The model under review builds one solid part; all positions refer to its coordinate system, in mm. A direction names the side the tool comes from. Coordinates: 2 decimals unless noted, no trailing zeros. Write each loop counter-clockwise with the first axis right and the second up, starting at its lowest first coordinate (ties: lowest second). Pieces come first, ordered by that corner, then holes. Notation, with made-up numbers: (-39, 49.25) - (-15, 49.25) arc R19 ccw to (-15, 83.25) - close; hole circle Ø9 at (7, 18.5). An arc over 180 degrees is marked (long way). Answer as CSV lines item,"result". Start each with the question number.
```python
from build123d import *

# Parameters (mm, degrees)
SKETCH_3_R          = 2.075
CUT_EXTRUDE_1_DEPTH = 60
FILLET_1_R          = 1


with BuildPart() as part:
    # 草图2 → 旋转1 (revolve)
    with BuildSketch(Plane.XY, mode=Mode.PRIVATE) as revolve_1_sk:
        Polygon((0, 0), (0, 50), (-15, 50), (-12, 25), (-15, 0), align=None)
    revolve(revolve_1_sk.sketch.rotate(Axis((0, 0, 0), (0, 1, 0)), 180), axis=Axis((0, 0, 0), (0, 1, 0)))

    # 草图3 → 切除-拉伸1 (cut)
    with BuildSketch(Plane.XZ):
        with Locations(Location((0, 0, 0), (0, 0, 270))):
            Circle(SKETCH_3_R)
    extrude(amount=-CUT_EXTRUDE_1_DEPTH, mode=Mode.SUBTRACT)

    # 圆角1
    fillet_1_edges = [part.edges().sort_by_distance(p)[0] for p in [
        (-15, 50, 0),
        (-15, 0, 0),
        (-12, 25, 0),
    ]]
    fillet(fillet_1_edges, radius=FILLET_1_R)


solid = part.part
```
(1) For pin 1 (10 mm diameter, centred on y = 11, z = 3.5, fed in from -X); pin 2 (1 mm diameter, centred on y = 34, z = -12, fed in from -X); pin 3 (1 mm diameter, centred on x = 3, y = 16.5, fed in from -Z); pin 4 (1 mm diameter, centred on x = -11.5, z = 7.5, fed in from -Y), all flat-tipped, find the tip position at first contact; note any pin that passes through.
(2) For faces 4 (the flat face through (3, 0, 0)), 5 (the conical face through (12.498, 34.193, -3.936)), list the 3-axis set-ups (+Z, -Z, +X, -X, +Y, -Y) from which the entire face can be reached by the end or side of a thin tool; tool diameter is ignored.
(3) The part is to be moulded in two halves that separate along X. For faces 1 (the cylindrical face through (-1.26, 24.65, 1.65)), 2 (the conical face through (12.536, 15.474, -3.948)), 3 (the flat face through (0, 50, 3)), say which applies: released by +X, released by -X, zero draft, split by the parting line, or undercut.
(4) Add section A-A on y = 14. Give the boundary of the cut face in (x, z) (3 decimals).
(5) Wall thickness on line 1 (X direction, y = 12, z = -0.75); line 2 (Z direction, x = -0.75, y = 19); line 3 (Z direction, x = 1.25, y = 18): over which ranges is each line inside the solid? List them lowest first.
(6) Add section B-B on y = 28.5. Give the boundary of the cut face in (x, z) (3 decimals), then the cut area to 3 significant figures.
Reported:
1,pin 1,"x = -14.16"
1,pin 2,"x = -6.24"
1,pin 3,"z = -12.8"
1,pin 4,"y = 0"
2,face 4,"+Z, -Z, +X, -X, -Y"
2,face 5,"none"
3,face 1,"undercut"
3,face 2,"split by the parting line"
3,face 3,"zero draft"
4,outline,"circle Ø26.64 at (0, 0); hole circle Ø4.15 at (0, 0)"
5,line 1,"-13.54 to -1.93, 1.93 to 13.54"
5,line 2,"-12.7 to -1.93, 1.93 to 12.7"
5,line 3,"-12.78 to -1.66, 1.66 to 12.78"
6,outline,"circle Ø24.84 at (0, 0); hole circle Ø4.15 at (0, 0)"
6,area,"471 mm²"
